Autodesk Inventor part; units mm, degrees
ref_plane "YZ Plane" through (0, 0, 0) normal (1, 0, 0) x (0, 1, 0)
ref_plane "XZ Plane" through (0, 0, 0) normal (0, 1, 0) x (-1, 0, 0)
ref_plane "XY Plane" through (0, 0, 0) normal (0, 0, 1) x (1, 0, 0)
sketch "Sketch1" plane through (0, 0, 0) normal (0, 0, 1) x (1, 0, 0)
  line L0 (-35.3, 51.65) -> (39.3, 51.65)
  line L1 (39.3, 51.65) -> (39.3, -36.65)
  line L2 (39.3, -36.65) -> (-35.3, -36.65)
  line L3 (-35.3, -36.65) -> (-35.3, 51.65)
  line L4 (-35.3, 51.65) -> (39.3, -36.65) construction
  line L5 (39.3, 51.65) -> (-35.3, -36.65) construction
  line L6 (34.3, 26.65) -> (-34.3, 26.65) construction
  line L7 (-34.3, 26.65) -> (-34.3, -26.65) construction
  line L8 (-34.3, -26.65) -> (34.3, -26.65) construction
  line L9 (34.3, -26.65) -> (34.3, 26.65) construction
  line L10 (34.3, 26.65) -> (-34.3, -26.65) construction
  line L11 (-34.3, 26.65) -> (34.3, -26.65) construction
  circle A0 centre (-20.3, 24.05) radius 1.6 construction
  circle A1 centre (-21.6, -24.15) radius 1.6 construction
  circle A2 centre (30.5, 8.85) radius 1.6 construction
  circle A3 centre (30.5, -19.05) radius 1.6 construction
  line L12 (-37.3, 53.65) -> (41.3, 53.65)
  line L13 (41.3, 53.65) -> (41.3, -38.65)
  line L14 (41.3, -38.65) -> (-37.3, -38.65)
  line L15 (-37.3, -38.65) -> (-37.3, 53.65)
  line L16 (-37.3, 53.65) -> (41.3, -38.65) construction
  line L17 (41.3, 53.65) -> (-37.3, -38.65) construction
  line L18 (30.5, 53.65) -> (30.5, -38.65) construction
  point P0 (0, 0)
  dimension "d82" = 6
  dimension "d0" = 53.3
  dimension "d2" = 68.6
  dimension "d3" = 14
  dimension "d4" = 2.5
  dimension "d5" = 50.8
  dimension "d6" = 27.9
  dimension "d7" = 5.1
  dimension "d8" = 3.2
  dimension "d9" = 25
  dimension "d10" = 1
  dimension "d11" = 2
  dimension "d12" = 2
  dimension "d59" = 5
  dimension "d62" = 10
  dimension "d63" = 2
  dimension "d64" = 2
  dimension "d92" = 15.2
  dimension "d94" = 1.3
extrude "Extrusion1" add sketch "Sketch1" against normal blind 2 contours L0 L1 L2 L3 | L12 L13 L14 L15
extrude "Extrusion2" add sketch "Sketch1" along normal blind 40
sketch "Sketch2" plane through (0, 0, 0) normal (0, 0, 1) x (1, 0, 0)
  circle A0 centre (-21.6, -24.15) radius 1.6 construction
  circle A1 centre (-20.3, 24.05) radius 4.15
  circle A2 centre (-21.6, -24.15) radius 4.15
  circle A3 centre (30.5, -19.05) radius 4.15
  circle A4 centre (30.5, 8.85) radius 4.15
  circle A5 centre (-20.3, 24.05) radius 2.15
  circle A6 centre (30.5, 8.85) radius 2.15
  circle A7 centre (-21.6, -24.15) radius 2.15
  circle A8 centre (30.5, -19.05) radius 2.15
  point P0 (0, 0)
  dimension "d17" = 8.3
  dimension "d19" = 4.3
extrude "Extrusion3" add sketch "Sketch2" along normal blind 5
sketch "Sketch7" plane through (0, 0, 0) normal (0, 0, 1) x (1, 0, 0)
  circle A0 centre (30.5, -19.05) radius 4.15
  circle A1 centre (30.5, 8.85) radius 4.15
  line L0 (-14.3, -17.05) -> (24.5, -17.05)
  line L1 (24.5, -17.05) -> (24.5, -21.05)
  line L2 (24.5, -21.05) -> (-14.3, -21.05)
  line L3 (-14.3, -21.05) -> (-14.3, -17.05)
  line L4 (-34.3, -26.65) -> (34.3, -26.65) construction
  line L5 (34.3, 26.65) -> (-34.3, 26.65) construction
  line L6 (34.3, -26.65) -> (34.3, 26.65) construction
  line L7 (-34.3, 26.65) -> (-34.3, -26.65) construction
  line L8 (24.5, 16.65) -> (-14.3, 16.65)
  line L9 (-14.3, 16.65) -> (-14.3, 12.65)
  line L10 (-14.3, 12.65) -> (24.5, 12.65)
  line L11 (24.5, 12.65) -> (24.5, 16.65)
  point P0 (0, 0)
  point P1 (24.5, -19.05)
  dimension "d79" = 4
  dimension "d80" = 20
  dimension "d81" = 6
  dimension "d82" = 6
  dimension "d83" = 20
  dimension "d86" = 10
  dimension "d87" = 0
extrude "Extrusion7" add sketch "Sketch7" along normal blind 8 contours L0 L1 L2 L3 | L11 L10 L9 L8
sketch "Sketch4" plane through (-37.3, -38.65, -2) normal (-1, 0, 0) x (0, 0, 1)
  line L0 (11.5, 56.3) -> (23.5, 56.3)
  line L1 (23.5, 56.3) -> (23.5, 43.3)
  line L2 (23.5, 43.3) -> (11.5, 43.3)
  line L3 (11.5, 43.3) -> (11.5, 56.3)
  line L4 (11.5, 56.3) -> (23.5, 43.3) construction
  line L5 (23.5, 56.3) -> (11.5, 43.3) construction
  line L6 (23.5, 15.25) -> (11.5, 15.25)
  line L7 (11.5, 15.25) -> (11.5, 25.25)
  line L8 (11.5, 25.25) -> (23.5, 25.25)
  line L9 (23.5, 25.25) -> (23.5, 15.25)
  line L10 (23.5, 15.25) -> (11.5, 25.25) construction
  line L11 (11.5, 15.25) -> (23.5, 25.25) construction
  line L12 (2, 0) -> (2, 92.3)
  line L13 (7, 58.55) -> (7, 66.85)
  line L14 (10, 21.6) -> (10, 17.6)
  line L15 (0, 92.3) -> (42, 92.3)
  line L16 (0, 0) -> (0, 92.3)
  line L17 (42, 0) -> (0, 0)
  line L18 (42, 92.3) -> (42, 0)
  point P0 (2, 38.65)
  point P1 (2, 65.3)
  point P2 (2, 65.3)
  point P3 (2, 65.3)
  point P4 (2, 12)
  point P5 (2, 12)
  point P6 (2, 12)
  point P7 (17.5, 49.8)
  point P8 (17.5, 20.25)
  point P9 (2, 107.3)
  dimension "d22" = 13
  dimension "d24" = 12
  dimension "d26" = 9
  dimension "d27" = 12
  dimension "d28" = 10
  dimension "d31" = 3.25
  dimension "d88" = 1.5
  dimension "d90" = 1.5
extrude "Extrusion4" cut sketch "Sketch4" against normal up to surface (2 mm away) contours L0 L1 L2 L3 | L6 L7 L8 L9
sketch "Sketch8" plane through (-37.3, 53.65, -2) normal (0, 1, 0) x (1, 0, 0)
  line L0 (15, -32) -> (15, -28.11) construction
  line L1 (11.9389, -28.11) -> (18.0611, -28.11)
  arc A0 (11.9389, -28.11) -> (18.0611, -28.11) centre (15, -32) ccw
  line L2 (78.6, -42) -> (78.6, 0) construction
  line L3 (0, 0) -> (78.6, 0) construction
  line L4 (0, 0) -> (0, -42) construction
  line L5 (78.6, -42) -> (0, -42) construction
  line L6 (78.6, -42) -> (78.6, 0) construction
  line L7 (78.6, -32) -> (0, -32) construction
  line L8 (0, 0) -> (0, -42) construction
  circle A1 centre (68.6, -32) radius 2.5
  circle A2 centre (58.6, -32) radius 2.5
  circle A3 centre (48.6, -32) radius 2.5
  circle A4 centre (38.6, -32) radius 2.5
  point P0 (37.3, -2)
  dimension "d97" = 9.9
  dimension "d98" = 3.89
  dimension "d99" = 10
  dimension "d100" = 15
  dimension "d101" = 5
  dimension "d104" = 10
  dimension "d109" = 10
extrude "Extrusion8" cut sketch "Sketch8" against normal up to next
properties part number "Arduino SMB-BNC box"
Source: CAD feature listing. Evaluate the final solid. Frame: model axes, mm. A direction names the side the tool comes from. Give positions to 0.01 mm unless a question says otherwise; leave off trailing zeros. Loops run counter-clockwise (first coordinate to the right, second up) from the corner with the lowest first, then second, coordinate; pieces in that order, holes last. Notation, with made-up numbers: (31.25, 13.25) -> (81.25, 13.25) arc R13 cw to (81.25, 28.25) -> close; hole circle Ø7 at (52, 12). An arc over 180 degrees is marked (long way). Use a Markdown table: item, result. Add a question column.
1) Line query: line 1 along X through (y, z) = (52.6, 30); line 2 along Y through (x, z) = (17.5, 32); line 3 along X through (y, z) = (-25.5, 38). Output: solid intervals per line, ascending. Write a range as [from, to].
2) First-contact query: pin 1 (3 mm diameter, centred on x = 4.5, y = 14.5, fed in from +Z); pin 2 (6.5 mm diameter, centred on x = 32.5, y = 7.5, fed in from +Z). Flat tips, straight axial feed; report the tip coordinate or a pass-through.
3) Section query C-C, the plane z = 12. Return the cut outline in (x, y).
4) Pull-direction query (Z, two-part tool) for faces 1 (the face through (-22, -24, 0)), 2 (the face through (32.55, -19.7, 2.46)), 3 (the face through (-22, 53, 26.11)); classes: +Z half, -Z half, draft (parallel to the pull), parting line (faces both ways), or undercut.
5) Section query A-A, the plane y = 8.85. Return the cut outline in (x, z).
6) Section query D-D, the plane y = 24.05. Return the cut outline in (x, z), then the cut area to 3 significant figures.
7) Section query B-B, the plane x = 11.3. Return the cut outline in (y, z).
8) Reachability of faces 4 (the face through (41.3, 8, 19)), 5 (the face through (-36, -23.4, 16)), 6 (the face through (-14.3, -19, 4)), 7 (the face through (0.97, 52.66, 27.52)) from +Z, -Z, +X, -X, +Y, -Y: full face, straight path, thin tool, end or side. Return the list, or none.
Numbers:
| question | item | result |
|---|---|---|
| 1 | line 1 | x = [-37.3, -27.25], [-17.35, -1.2], [3.8, 8.8], [13.8, 18.8], [23.8, 28.8], [33.8, 41.3] |
| 1 | line 2 | y = [-38.65, -36.65], [51.65, 53.65] |
| 1 | line 3 | x = [-37.3, -35.3], [39.3, 41.3] |
| 2 | pin 1 | stops at z = 8 |
| 2 | pin 2 | stops at z = 5 |
| 3 | outline | (-37.3, -38.65) -> (41.3, -38.65) -> (41.3, 53.65) -> (-37.3, 53.65) -> (-37.3, 17.65) -> (-35.3, 17.65) -> (-35.3, 51.65) -> (39.3, 51.65) -> (39.3, -36.65) -> (-35.3, -36.65) -> (-35.3, -23.4) -> (-37.3, -23.4) -> close; (-37.3, -13.4) -> (-35.3, -13.4) -> (-35.3, 4.65) -> (-37.3, 4.65) -> close |
| 4 | face 1 | +Z half |
| 4 | face 2 | draft |
| 4 | face 3 | undercut |
| 5 | outline | (-37.3, -2) -> (41.3, -2) -> (41.3, 40) -> (39.3, 40) -> (39.3, 0) -> (34.65, 0) -> (34.65, 5) -> (32.65, 5) -> (32.65, 0) -> (28.35, 0) -> (28.35, 5) -> (26.35, 5) -> (26.35, 0) -> (-35.3, 0) -> (-35.3, 9.5) -> (-37.3, 9.5) -> close; (-37.3, 21.5) -> (-35.3, 21.5) -> (-35.3, 40) -> (-37.3, 40) -> close |
| 6 | outline | (-37.3, -2) -> (41.3, -2) -> (41.3, 40) -> (39.3, 40) -> (39.3, 0) -> (-16.15, 0) -> (-16.15, 5) -> (-18.15, 5) -> (-18.15, 0) -> (-22.45, 0) -> (-22.45, 5) -> (-24.45, 5) -> (-24.45, 0) -> (-35.3, 0) -> (-35.3, 40) -> (-37.3, 40) -> close |
| 6 | area | 337 mm2 |
| 7 | outline | (-38.65, -2) -> (53.65, -2) -> (53.65, 27.5) -> (51.65, 27.5) -> (51.65, 0) -> (16.65, 0) -> (16.65, 8) -> (12.65, 8) -> (12.65, 0) -> (-17.05, 0) -> (-17.05, 8) -> (-21.05, 8) -> (-21.05, 0) -> (-36.65, 0) -> (-36.65, 40) -> (-38.65, 40) -> close; (51.65, 32.5) -> (53.65, 32.5) -> (53.65, 40) -> (51.65, 40) -> close |
| 8 | face 4 | +Z, -Z, +X, +Y, -Y |
| 8 | face 5 | -X |
| 8 | face 6 | +Z |
| 8 | face 7 | +Y |
